from build123d import *

# Parameters (mm, degrees)
F0_W     = 76.2
F0_H     = 76.2
F1_DEPTH = 76.2
F3_DEPTH = 76.201
F4_W     = 25.4
F4_H     = 25.4
F5_DEPTH = 12.7


with BuildPart() as f1:
    # F0 (on Top) → F1 (new body)
    with BuildSketch(Plane.XY):
        with Locations((-33.296083, 29.620429)):
            Rectangle(F0_W, F0_H)
    extrude(amount=F1_DEPTH)

    # F2 (on face) → F3 (cut, through all)
    with BuildSketch(Plane.XY.offset(76.2)):
        Polygon((-22.887098, 0), (-1.908828, 30.366746), (-24.306678, 59.702107), (-59.12758, 47.465611), (-58.250232, 10.56768), align=None)
    extrude(amount=-F3_DEPTH, mode=Mode.SUBTRACT)

    # F4 (on face) → F5 (cut)
    with BuildSketch(Plane.XZ.offset(8.479571)):
        with Locations((-33.296083, 38.1)):
            Rectangle(F4_W, F4_H)
    extrude(amount=-F5_DEPTH, mode=Mode.SUBTRACT)


solid = f1.part
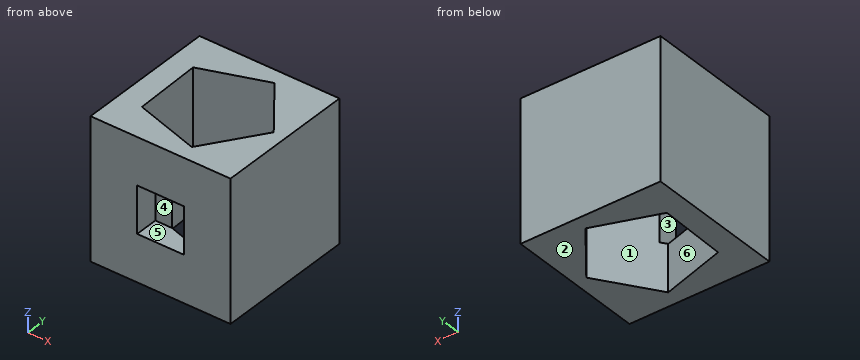
Geometry check sheet. Reference: the model listing, model coordinates, mm. Face numbers are marked on the shaded views. A direction names the side the tool comes from. Round coordinates to 2 decimals unless told otherwise and drop trailing zeros. Loops run counter-clockwise (first coordinate to the right, second up) from the corner with the lowest first, then second, coordinate; pieces in that order, holes last.
Item 1: Gauge pin test, flat ends, axial feed: pin 1 (6 mm diameter, centred on x = -27.5, y = 55, fed in from +Z); pin 2 (10 mm diameter, centred on x = -29, y = -5, fed in from -Z); pin 3 (2.5 mm diameter, centred on x = -42, z = 39, fed in from -Y). Record the tip position at first contact, or that the pin passes through.
Item 2: Cross-section at C-C on x = -13.5. Record the boundary of the cut face in (y, z), then the cut area to 3 significant figures.
Item 3: Cross-section at A-A on z = 18.5. Record the boundary of the cut face in (x, y).
Item 4: Thickness scan on line 1 (Z direction, x = -35.5, y = 3.5); line 2 (X direction, y = 0, z = 45); line 3 (X direction, y = 19.5, z = 63.5). Record the ranges inside material, lowest first.
Item 5: Mould release check, pull along Y, two halves, no side actions. Record for the marked faces 4, 5 and 6: pulls with the +Y half, pulls with the -Y half, needs draft (parallel to the pull), parting line crosses it, or undercut.
Item 6: Access from +Z, -Z, +X, -X, +Y, -Y to the whole of each face (thin tool, end or side, straight path). Record for the marked faces 1, 2 and 3.
Item 7: Cross-section at D-D on z = 29.5. Record the boundary of the cut face in (x, y).
Item 8: Cross-section at B-B on y = 22.5. Record the boundary of the cut face in (x, z).
Answer sheet:
1. pin 1: passes through
1. pin 2: stops at z = 0
1. pin 3: stops at y = 4.22
2. outline: (-8.48, 0) - (13.59, 0) - (13.59, 76.2) - (-8.48, 76.2) - close; (45.55, 0) - (67.72, 0) - (67.72, 76.2) - (45.55, 76.2) - close
2. area: 3,370 mm2
3. outline: (-71.4, -8.48) - (4.8, -8.48) - (4.8, 67.72) - (-71.4, 67.72) - close; hole (-59.13, 47.47) - (-58.25, 10.57) - (-22.89, 0) - (-1.91, 30.37) - (-24.31, 59.7) - close
4. line 1: z = 0 to 25.4, 50.8 to 76.2
4. line 2: x = -71.4 to -46, -20.6 to 4.8
4. line 3: x = -71.4 to -58.46, -9.42 to 4.8
5. face 4: pulls with the -Y half
5. face 5: needs draft
5. face 6: undercut
6. face 1: +Z, -Z
6. face 2: -Z, +X, -X, +Y, -Y
6. face 3: -Y
7. outline: (-71.4, -8.48) - (-46, -8.48) - (-46, 4.22) - (-37.01, 4.22) - (-58.25, 10.57) - (-59.13, 47.47) - (-24.31, 59.7) - (-1.91, 30.37) - (-20.6, 3.32) - (-20.6, -8.48) - (4.8, -8.48) - (4.8, 67.72) - (-71.4, 67.72) - close
8. outline: (-71.4, 0) - (-58.53, 0) - (-58.53, 76.2) - (-71.4, 76.2) - close; (-7.34, 0) - (4.8, 0) - (4.8, 76.2) - (-7.34, 76.2) - close
